Part model, mm, in its own coordinate system. Round coordinates to 2 decimals unless told otherwise and drop trailing zeros. Order: outer loops, then holes, each group sorted by start corner. A loop starts at its lowest first (then second) coordinate and runs counter-clockwise, first axis right, second up. Notation, with made-up numbers: M 45.5,16.25 L 74.5,16.25 A24 ccw 74.5,42.25 Z; hole C 88,-38.5 d9. An arc over 180 degrees is marked long. Write each question's results on one line, items separated by ' | '. Start each with the question number.
1. Band-saw the part on C-C, the plane x = 180. List the corners of the cut face in (y, z), then the cut area to 3 significant figures.
2. Band-saw the part on B-B, the plane y = 2.75. List the corners of the cut face in (x, z), then the cut area to 3 significant figures.
3. Drop a flat-ended pin along its axis: pin 1 Ø3.5 at (x, z) = (-155.25, 0) entering from -Y. Give the stop position or say it passes through.
4. Band-saw the part on A-A, the plane x = 0. List the corners of the cut face in (y, z).
5. Two-plate mould, pull along X, no slides. Class faces 1 (the face through (172.564, 5.916, 0.976)), 2 (the face through (-3, 0, -7)), 3 (the face through (200, 6, 0)): +X half, -X half, draft (parallel to the pull), parting line (faces both ways), or undercut.
6. Probe L1, parallel to X at y = 7.25, z = 0; L2, parallel to Z at x = -187.25, y = 8.5; L3, parallel to X at y = 11, z = 3. List the from-to ranges inside material, lowest first. Write a range as [from, to].
```python
from build123d import *

# Parameters (mm, degrees)
SKETCH1_W           = 400
SKETCH1_H           = 30
SKETCH1_R           = 5
SKETCH1_R_2         = 2.75
BOSS_EXTRUDE1_DEPTH = 12
SKETCH2_R           = 7.5
CUT_EXTRUDE1_DEPTH  = 20


with BuildPart() as part:
    # Sketch1 → Boss-Extrude1 (new body)
    with BuildSketch(Plane(origin=(0, 0, 0), x_dir=(1, 0, 0), z_dir=(0, 1, 0))):
        Rectangle(SKETCH1_W, SKETCH1_H)
        with Locations(Location((0, 0, 0), (0, 0, 270))):
            Circle(SKETCH1_R, mode=Mode.SUBTRACT)
        with Locations(Location((-187.25, 0, 0), (0, 0, 270))):
            Circle(SKETCH1_R_2, mode=Mode.SUBTRACT)
        with Locations(Location((-155.25, 0, 0), (0, 0, 270))):
            Circle(SKETCH1_R_2, mode=Mode.SUBTRACT)
    extrude(amount=BOSS_EXTRUDE1_DEPTH)

    # Sketch2 → Cut-Extrude1 (cut)
    with BuildSketch(Plane(origin=(0, 0, 0), x_dir=(1, 0, 0), z_dir=(0, 1, 0))):
        with Locations(Location((155, 0, 0), (0, 0, 90))):
            Circle(SKETCH2_R)
        with Locations(Location((180, 0, 0), (0, 0, 90))):
            Circle(SKETCH2_R)
    extrude(amount=CUT_EXTRUDE1_DEPTH, mode=Mode.SUBTRACT)


solid = part.part
```
Solution:
1) outline: M 0,-15 L 12,-15 L 12,-7.5 L 0,-7.5 Z; M 0,7.5 L 12,7.5 L 12,15 L 0,15 Z | area: 180 mm^2
2) outline: M -200,-15 L 200,-15 L 200,15 L -200,15 Z; hole C -187.25,0 d5.5; hole C -155.25,0 d5.5; hole C 0,0 d10; hole C 155,0 d15; hole C 180,0 d15 | area: 11,500 mm^2
3) pin 1: through
4) outline: M 0,-15 L 12,-15 L 12,-5 L 0,-5 Z; M 0,5 L 12,5 L 12,15 L 0,15 Z
5) face 1: undercut | face 2: draft | face 3: +X half
6) L1: [-200, -190], [-184.5, -158], [-152.5, -5], [5, 147.5], [162.5, 172.5], [187.5, 200] | L2: [-15, -2.75], [2.75, 15] | L3: [-200, -4], [4, 148.13], [161.87, 173.13], [186.87, 200]
